from build123d import *

# Parameters (mm, degrees)
F0_R     = 5
F0_R_2   = 4
F1_DEPTH = 600
F3_D     = 6
F3_DEPTH = 5.001
F4_D     = 6


with BuildPart() as f1:
    # F0 (on Top) → F1 (new body)
    with BuildSketch(Plane.XY):
        Circle(F0_R)
        Circle(F0_R_2, mode=Mode.SUBTRACT)
    extrude(amount=F1_DEPTH)

    # F3 (through all, one way)
    with BuildSketch(Plane(origin=(0, 0, 0), x_dir=(1, 0, 0), z_dir=(0, 1, 0))):
        with Locations((0, -6), (0, -594)):
            Circle(F3_D / 2)
    extrude(amount=-F3_DEPTH, mode=Mode.SUBTRACT)

    # F4 (through all)
    with Locations(Plane.XZ):
        with Locations((0, 594), (0, 6)):
            Hole(F4_D / 2)


solid = f1.part
Could you check a few things on this model? Use its own coordinates, in mm. Coordinates: 2 decimals unless noted, no trailing zeros. Order: outer loops, then holes, each group sorted by start corner. A loop starts at its lowest first (then second) coordinate and runs counter-clockwise, first axis right, second up.
Q1. Suppose I cut it at A-A on x = 0. Please give me the cut outline in (y, z).
Q2. Suppose I cut it at C-C on z = 310.5. Please give me the cut outline in (x, y), and give its area (3 significant figures).
Q3. Please list where these lines run through material, in increasing order: L1, parallel to Z at x = 0, y = -4.3; L2, parallel to Y at x = 0.25, z = 547.5; L3, parallel to X at y = 0.5, z = 104.
Q4. Suppose I cut it at B-B on y = 0. Please give me the cut outline in (x, z).
Answer:
1. outline: (-5, 0) - (-4, 0) - (-4, 3) - (-5, 3) - close; (-5, 9) - (-4, 9) - (-4, 591) - (-5, 591) - close; (-5, 597) - (-4, 597) - (-4, 600) - (-5, 600) - close; (4, 0) - (5, 0) - (5, 3) - (4, 3) - close; (4, 9) - (5, 9) - (5, 591) - (4, 591) - close; (4, 597) - (5, 597) - (5, 600) - (4, 600) - close
2. outline: circle Ø10 at (0, 0); hole circle Ø8 at (0, 0)
2. area: 28.3 mm2
3. L1: z = 0 to 3, 9 to 591, 597 to 600
3. L2: y = -4.99 to -3.99, 3.99 to 4.99
3. L3: x = -4.97 to -3.97, 3.97 to 4.97
4. outline: (-5, 0) - (-4, 0) - (-4, 600) - (-5, 600) - close; (4, 0) - (5, 0) - (5, 600) - (4, 600) - close
